Can you work these out from the model? Positions are in its coordinate system, mm. Face numbers are marked on the shaded views. A direction names the side the tool comes from. Round coordinates to 2 decimals unless told otherwise and drop trailing zeros. Loops run counter-clockwise (first coordinate to the right, second up) from the corner with the lowest first, then second, coordinate; pieces in that order, holes last. Notation, with made-up numbers: M -39,5 L 3,5 A22 cw 3,24 Z; hole C 21.5,-16.75 d7. An arc over 180 degrees is marked long. Answer as CSV lines item,"result".
from build123d import *

# Parameters (mm, degrees)
SKETCH1_W           = 42.5
SKETCH1_H           = 42.5
SKETCH1_R           = 14
BOSS_EXTRUDE1_DEPTH = 4
CUT_EXTRUDE1_DEPTH  = 10
SKETCH3_W           = 31.186291502
SKETCH3_H           = 44.5
BOSS_EXTRUDE2_DEPTH = 4
SKETCH4_W           = 31.186291502
SKETCH4_H           = 44.5
BOSS_EXTRUDE3_DEPTH = 4
BOSS_EXTRUDE5_DEPTH = 4
SKETCH8_W           = 31.186291502
SKETCH8_H           = 80
BOSS_EXTRUDE6_DEPTH = 4


with BuildPart() as part:
    # Sketch1 → Boss-Extrude1 (new body)
    with BuildSketch(Plane(origin=(0, 0, 0), x_dir=(0, 1, 0), z_dir=(0, 0, 1))):
        Rectangle(SKETCH1_W, SKETCH1_H)
        with Locations(Location((0, 0, 0), (0, 0, 270))):
            Circle(SKETCH1_R, mode=Mode.SUBTRACT)
    extrude(amount=BOSS_EXTRUDE1_DEPTH)

    # Sketch2 → Cut-Extrude1 (cut)
    with BuildSketch(Plane.XY.offset(4)):
        Polygon((-15.593145751, 21.25), (-21.25, 15.593145751), (-21.25, 21.25), align=None)
        Polygon((-21.25, -15.593145751), (-15.593145751, -21.25), (-21.25, -21.25), align=None)
        Polygon((15.593145751, -21.25), (21.25, -15.593145751), (21.25, -21.25), align=None)
        Polygon((15.593145751, 21.25), (21.25, 15.593145751), (21.25, 21.25), align=None)
    extrude(amount=-CUT_EXTRUDE1_DEPTH, mode=Mode.SUBTRACT)

    # Sketch3 → Boss-Extrude2 (add)
    with BuildSketch(Plane(origin=(-21.25, 0, 0), x_dir=(0, -1, 0), z_dir=(-1, 0, 0))):
        with Locations((0, -18.25)):
            Rectangle(SKETCH3_W, SKETCH3_H)
    extrude(amount=BOSS_EXTRUDE2_DEPTH)

    # Sketch4 → Boss-Extrude3 (add)
    with BuildSketch(Plane.YZ.offset(21.25)):
        with Locations((0, -18.25)):
            Rectangle(SKETCH4_W, SKETCH4_H)
    extrude(amount=BOSS_EXTRUDE3_DEPTH)

    # Sketch6 → Boss-Extrude5 (add)
    with BuildSketch(Plane(origin=(0, 0, -40.5), x_dir=(1, 0, 0), z_dir=(0, 0, -1))):
        Polygon((-21.25, 15.593145751), (-25.25, 15.593145751), (-25.25, -15.593145751), (-21.25, -15.593145751), (-15.593145751, -21.25), (15.593145751, -21.25), (21.25, -15.593145751), (25.25, -15.593145751), (25.25, 15.593145751), (21.25, 15.593145751), (15.593145751, 21.25), (-15.593145751, 21.25), align=None)
    extrude(amount=BOSS_EXTRUDE5_DEPTH)

    # Sketch8 → Boss-Extrude6 (add)
    with BuildSketch(Plane.XY.offset(4)):
        with Locations((0, -61.25)):
            Rectangle(SKETCH8_W, SKETCH8_H)
    extrude(amount=-BOSS_EXTRUDE6_DEPTH)


solid = part.part
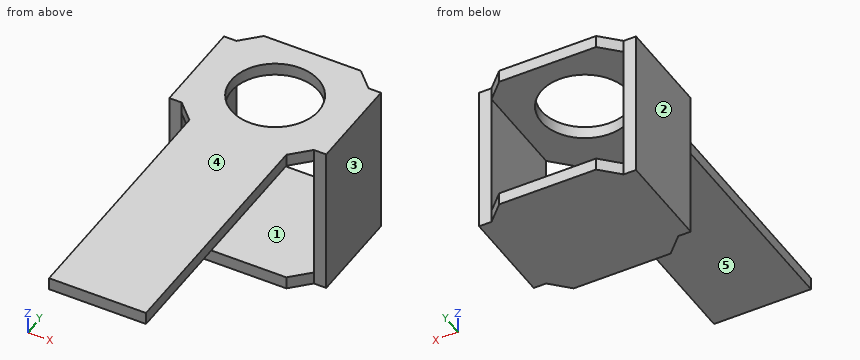
Item 1: On a 3-axis mill with a long thin cutter (end or side, diameter ignored), from which of +Z, -Z, +X, -X, +Y, -Y can I reach the whole of each face in a straight line? I mean the marked faces 1 and 2. Say none if no direction works.
Output:
face 1,"+Y, -Y"
face 2,"+Z, -Z, -X, +Y, -Y"
Item 2: If I drill on line 1 along X through (y, z) = (6, -22.5); line 2 along Y through (x, z) = (0, 1.5); line 3 along Z through (x, y) = (10.5, -21), over which ranges is the centre line in solid material (lowest first)? Write a range as from..to.
Output:
line 1,"x = -25.25..-21.25, 21.25..25.25"
line 2,"y = -101.25..-14, 14..21.25"
line 3,"z = -44.5..-40.5, 0..4"
Item 3: If we section it at D-D on y = 0: Write out the boundary of the cut face in (x, z), then the cut area to 3 significant figures.
Output:
outline,"M -25.25,-44.5 L 25.25,-44.5 L 25.25,4 L 14,4 L 14,0 L 21.25,0 L 21.25,-40.5 L -21.25,-40.5 L -21.25,0 L -14,0 L -14,4 L -25.25,4 Z"
area,"616 mm2"
Item 4: If we section it at C-C on y = -20: Write out the boundary of the cut face in (x, z), then the cut area to 3 significant figures.
Output:
outline,"M -16.84,-44.5 L 16.84,-44.5 L 16.84,-40.5 L -16.84,-40.5 Z; M -16.84,0 L 16.84,0 L 16.84,4 L -16.84,4 Z"
area,"269 mm2"
Item 5: If we section it at A-A on z = -38.5: Write out the boundary of the cut face in (x, y), then the cut area to 3 significant figures.
Output:
outline,"M -25.25,-15.59 L -21.25,-15.59 L -21.25,15.59 L -25.25,15.59 Z; M 21.25,-15.59 L 25.25,-15.59 L 25.25,15.59 L 21.25,15.59 Z"
area,"249 mm2"
Item 6: We'd pull the mould along X, two halves only. Please class the marked faces 3, 4 and 5: released by +X, released by -X, zero draft, split by the parting line, or undercut.
Output:
face 3,"released by +X"
face 4,"zero draft"
face 5,"undercut"
Item 7: If we section it at B-B on x = 0: Write out the boundary of the cut face in (y, z).
Output:
outline,"M -101.25,0 L -14,0 L -14,4 L -101.25,4 Z; M -21.25,-44.5 L 21.25,-44.5 L 21.25,-40.5 L -21.25,-40.5 Z; M 14,0 L 21.25,0 L 21.25,4 L 14,4 Z"
Item 8: Will these pins go through, and if not, where does the flat tip stop? pin 1 (4.5 mm diameter, centred on y = -77, z = 1.5, fed in from +X); pin 2 (1.2 mm diameter, centred on x = 0, z = -42, fed in from -Y); pin 3 (1.2 mm diameter, centred on y = -48.5, z = 1.5, fed in from -X); pin 4 (21 mm diameter, centred on x = -8.5, y = -7, fed in from +Z).
Output:
pin 1,"stops at x = 15.59"
pin 2,"stops at y = -21.25"
pin 3,"stops at x = -15.59"
pin 4,"stops at z = 4"
